from build123d import *

# Parameters (mm, degrees)
F1_DEPTH = 90
F2_R     = 5


with BuildPart() as f1:
    # F0 (on Top) → F1 (new body)
    with BuildSketch(Plane.XY):
        Polygon((-125.3208518028, 0), (0, 0), (0, 60.1540058851), (-94.9204340577, 60.1540058851), align=None)
    extrude(amount=F1_DEPTH)

    # F2
    f2_edges = [f1.edges().sort_by_distance(p)[0] for p in [
        (-47.460217, 60.154006, 90),
        (0, 30.077003, 90),
        (-62.660426, 0, 90),
        (-110.120643, 30.077003, 90),
        (0, 60.154006, 45),
        (0, 0, 45),
        (-94.920434, 60.154006, 45),
        (-125.320852, 0, 45),
        (-110.120643, 30.077003, 0),
        (-62.660426, 0, 0),
        (-47.460217, 60.154006, 0),
        (0, 30.077003, 0),
    ]]
    fillet(f2_edges, radius=F2_R)

    # F1_face (on face) → F3 (revolve)
    with BuildSketch(Plane(origin=(-55.0281837539, 29.0125128526, 90), x_dir=(1, 0, 0), z_dir=(0, 0, 1))):
        Polygon((50.0281837539, 26.1414930325), (-36.8168888954, 26.1414930325), (-62.1635421741, -24.0125128526), (50.0281837539, -24.0125128526), align=None)
    revolve(axis=Axis((-61.095862964, 0, 85), (1, 0, 0)))


solid = f1.part
CAD build for the part. Positions are in the model's coordinates, mm. A direction names the side the tool comes from. Round coordinates to 2 decimals unless told otherwise and drop trailing zeros. Write each loop counter-clockwise with the first axis right and the second up, starting at its lowest first coordinate (ties: lowest second). Pieces come first, ordered by that corner, then holes. Notation, with made-up numbers: (63.5, -18.5) -> (103.5, -18.5) arc R30 ccw to (103.5, 4.5) -> close; hole circle Ø3 at (-24.5, 88.25). An arc over 180 degrees is marked (long way). Answer as a JSON object with one key per item and string values.
(1) Two-plate mould, pull along Y, no slides. Class faces 1 (the face through (-60.31, -6.46, 87.88)), 2 (the face through (-107.9, 31.3, 88.5)), 3 (the face through (-5, -6, 92)): +Y half, -Y half, draft (parallel to the pull), parting line (faces both ways), or undercut.
Reported:
{"face 1": "undercut", "face 2": "+Y half", "face 3": "draft"}
(2) Pin check, flat tips, straight feed: P1, Ø5, axis at y = -3.5, z = 54, coming from the +X side; P2, Ø6, axis at x = -68, y = -25.5, coming from the -Z side; P3, Ø1.5, axis at y = -0.5, z = 99.5, coming from the -X side. Stop position of each tip, or through.
Reported:
{"P1": "stops at x = -5", "P2": "stops at z = 34.4", "P3": "stops at x = -113.24"}
(3) Band-saw the part on A-A, the plane x = -17. List the corners of the cut face in (y, z), then the cut area to 3 significant figures.
Reported:
{"outline": "(0, 5) arc R5 ccw to (5, 0) -> (55.15, 0) arc R5 ccw to (60.15, 5) -> (60.15, 85) arc R5 ccw to (55.15, 90) arc R55.38 ccw (long way) to (0, 29.62) -> close; hole (0, 77.93) -> (0, 85) arc R5 cw to (5, 90) arc R7.07 ccw (long way) to start", "area": "12,300 mm^2"}
(4) Which spindle directions (+Z, -Z, +X, -X, +Y, -Y) get a long thin tool onto all of the face, cutting with end or side? Do faces 4 (the face through (-62, 0, 81)), 5 (the face through (-2, 1, 46)), 6 (the face through (-74, 0, 25)). Say none if no direction does.
Reported:
{"face 4": "+X, -X", "face 5": "+Z, -Z, +X, -Y", "face 6": "-Z, -X, -Y"}
(5) Probe probe 1 along Y at (x, z) = (-28, 85); probe 2 along Z at (x, y) = (-16.5, 1.5); probe 3 along Y at (x, z) = (-81, 10). List the from-to ranges inside material, lowest first. Write a range as [from, to].
Reported:
{"probe 1": "y = [-55.38, -7.07], [0, 60.15]", "probe 2": "z = [1.43, 88.57], [91.91, 140.36]", "probe 3": "y = [0, 60.15]"}
(6) Band-saw the part on B-B, the plane z = 22. List the corners of the cut face in (x, y), then the cut area to 3 significant figures.
Reported:
{"outline": "(-121.65, 7.26) arc R5 ccw to (-117.19, 0) -> (-5, 0) arc R5 ccw to (0, 5) -> (0, 55.15) arc R5 ccw to (-5, 60.15) -> (-91.85, 60.15) arc R5 ccw to (-96.31, 57.41) -> close", "area": "6,600 mm^2"}
